Input: part model. Units: mm. Frame: model coordinates. A direction names the side the tool comes from. Give positions to 0.01 mm unless a question says otherwise; leave off trailing zeros. Loops run counter-clockwise (first coordinate to the right, second up) from the corner with the lowest first, then second, coordinate; pieces in that order, holes last. Notation, with made-up numbers: M -7,-35 L 11,-35 A15 ccw 11,-9 Z; hole C -25,-24 d7. An arc over 180 degrees is marked long. One line per item, written item: value. Start each with the question number.
(1) Pin query (flat end, axial travel): P1, Ø1.5, axis at x = 0.5, y = -0.5, coming from the +Z side; P2, Ø1, axis at y = 2.5, z = -1.5, coming from the +X side; P3, Ø1.5, axis at x = 2.5, z = 0, coming from the +Y side. Return the tip coordinate at first contact, or that it passes through.
(2) Section C-C on z = -2.25. Output: boundary loops of the cut face in (x, y), plus the area to 3 significant figures.
(3) Section A-A on z = 2.25. Output: boundary loops of the cut face in (x, y), plus the area to 3 significant figures.
(4) Section B-B on x = 0. Output: boundary loops of the cut face in (y, z), plus the area to 3 significant figures.
(5) Pull-direction query (X, two-part tool) for faces 4 (the flat face through (-1.289, 0.766, 2.514)), 5 (the cylindrical face through (3.233, 1.341, 1.578)), 6 (the flat face through (0, 0, -12)); classes: released by +X, released by -X, zero draft, split by the parting line, or undercut.
(6) Access query for faces 1 (the flat face through (-1.5, -0.7, 3.5)), 2 (the flat face through (-1.31, -0.73, 2.51)), 3 (the cylindrical face through (0.54, 2.44, -5.92)). Directions: +Z, -Z, +X, -X, +Y, -Y. A direction counts if a zero-diameter tool reaches every point of the face in a straight line with its end or side. Return the directions, or none.
(7) Ray query, line 1 along Z through (x, y) = (-0.5, 3); line 2 along Y through (x, z) = (1, 1); line 3 along Y through (x, z) = (0.75, -1). Return the intervals inside material, ascending. Write a range as from..to.
Autodesk Inventor part; units mm, degrees
ref_plane "YZ Plane" through (0, 0, 0) normal (1, 0, 0) x (0, 1, 0)
ref_plane "XZ Plane" through (0, 0, 0) normal (0, 1, 0) x (-1, 0, 0)
ref_plane "XY Plane" through (0, 0, 0) normal (0, 0, 1) x (1, 0, 0)
sketch "Sketch1" plane through (0, 0, 0) normal (0, 0, 1) x (1, 0, 0)
  circle A0 centre (0, 0) radius 3.5
  dimension "d0" = 7
extrude "Extrusion1" add sketch "Sketch1" along normal blind 3.5
sketch "Sketch2" plane through (0, 0, 0) normal (0, 0, -1) x (-1, 0, 0)
  circle A0 centre (0, 0) radius 2.5
  dimension "d3" = 5
extrude "Extrusion2" add sketch "Sketch2" along normal blind 12
sketch "Sketch3" plane through (0, 0, 3.5) normal (0, 0, 1) x (1, 0, 0)
  circle A0 centre (0, 0) radius 3.5
  line L0 (-0.8347, 1.5177) -> (0.897, 1.4817)
  line L1 (0.897, 1.4817) -> (1.7317, -0.0359)
  line L2 (1.7317, -0.0359) -> (0.8347, -1.5177)
  line L3 (0.8347, -1.5177) -> (-0.897, -1.4817)
  line L4 (-0.897, -1.4817) -> (-1.7317, 0.0359)
  line L5 (-1.7317, 0.0359) -> (-0.8347, 1.5177)
  dimension "d6" = 3
extrude "Extrusion3" cut sketch "Sketch3" against normal blind 2 contours L0 L1 L2 L3 L4 L5
thread "Thread1"
chamfer "Chamfer1" distance 0.3 angle 45 1 edges at (-3.5, 0, 3.5)
properties part number "M5 Cap Head Screw"
Output values:
1. P1: stops at z = 1.5
1. P2: stops at x = 1.5
1. P3: stops at y = 3.03
2. outline: C 0,0 d5
2. area: 19.6 mm²
3. outline: C 0,0 d7; hole M -1.73,0.04 L -0.9,-1.48 L 0.83,-1.52 L 1.73,-0.04 L 0.9,1.48 L -0.83,1.52 Z
3. area: 30.7 mm²
4. outline: M -3.5,0 L -2.5,0 L -2.5,-12 L 2.5,-12 L 2.5,0 L 3.5,0 L 3.5,3.2 L 3.2,3.5 L 1.5,3.5 L 1.5,1.5 L -1.5,1.5 L -1.5,3.5 L -3.2,3.5 L -3.5,3.2 Z
4. area: 78.4 mm²
5. face 4: undercut
5. face 5: split by the parting line
5. face 6: zero draft
6. face 1: +Z, +X, -X, +Y, -Y
6. face 2: +Z
6. face 3: -Z
7. line 1: z = 0..3.5
7. line 2: y = -3.35..3.35
7. line 3: y = -2.38..2.38
